```python
from build123d import *

# Parameters (mm, degrees)
SKETCH1_R           = 2.413
BOSS_EXTRUDE1_DEPTH = 3.175
FILLET1_R           = 6.35


with BuildPart() as part:
    # Sketch1 → Boss-Extrude1 (new body)
    with BuildSketch(Plane.XY):
        Polygon((-76.2, 0), (76.2, 0), (76.2, -50.8), (25.4, -50.8), (25.4, -101.6), (-25.4, -101.6), (-25.4, -50.8), (-76.2, -50.8), align=None)
        with Locations((-63.5, -12.7)):
            Circle(SKETCH1_R, mode=Mode.SUBTRACT)
        with Locations((-63.5, -38.1)):
            Circle(SKETCH1_R, mode=Mode.SUBTRACT)
        with Locations((-38.1, -12.7)):
            Circle(SKETCH1_R, mode=Mode.SUBTRACT)
        with Locations((-38.1, -38.1)):
            Circle(SKETCH1_R, mode=Mode.SUBTRACT)
        with Locations((-12.7, -88.9)):
            Circle(SKETCH1_R, mode=Mode.SUBTRACT)
        with Locations((-12.7, -63.5)):
            Circle(SKETCH1_R, mode=Mode.SUBTRACT)
        with Locations(Location((12.7, -88.9, 0), (0, 0, 180))):
            Circle(SKETCH1_R, mode=Mode.SUBTRACT)
        with Locations(Location((12.7, -63.5, 0), (0, 0, 180))):
            Circle(SKETCH1_R, mode=Mode.SUBTRACT)
        with Locations(Location((63.5, -38.1, 0), (0, 0, 180))):
            Circle(SKETCH1_R, mode=Mode.SUBTRACT)
        with Locations(Location((38.1, -38.1, 0), (0, 0, 180))):
            Circle(SKETCH1_R, mode=Mode.SUBTRACT)
        with Locations(Location((38.1, -12.7, 0), (0, 0, 180))):
            Circle(SKETCH1_R, mode=Mode.SUBTRACT)
        with Locations(Location((63.5, -12.7, 0), (0, 0, 180))):
            Circle(SKETCH1_R, mode=Mode.SUBTRACT)
    extrude(amount=BOSS_EXTRUDE1_DEPTH)

    # Fillet1
    fillet1_edges = [part.edges().sort_by_distance(p)[0] for p in [
        (25.4, -101.6, 1.5875),
        (-25.4, -101.6, 1.5875),
        (-25.4, -50.8, 1.5875),
        (-76.2, -50.8, 1.5875),
        (-76.2, 0, 1.5875),
        (76.2, 0, 1.5875),
        (76.2, -50.8, 1.5875),
        (25.4, -50.8, 1.5875),
    ]]
    fillet(fillet1_edges, radius=FILLET1_R)


solid = part.part
```
The model under review builds one solid part; all positions refer to its coordinate system, in mm. A direction names the side the tool comes from. Round coordinates to 2 decimals unless told otherwise and drop trailing zeros. Loops run counter-clockwise (first coordinate to the right, second up) from the corner with the lowest first, then second, coordinate; pieces in that order, holes last. Notation, with made-up numbers: (76, -1.5) -> (108, -1.5) arc R32 ccw to (108, 28.5) -> close; hole circle Ø8 at (24, 89.25). An arc over 180 degrees is marked (long way). Answer in a Markdown table with one row per item.
1) Tool access review of faces 1 (the flat face through (-25.4, -76, 2)), 2 (the cylindrical face through (39.88, -39.73, 1.57)): name each direction out of +Z, -Z, +X, -X, +Y, -Y from which nothing blocks a thin tool from reaching the whole face with its end or side.
Taken from the geometry:
| item | result |
|---|---|
| face 1 | +Z, -Z, -X, -Y |
| face 2 | +Z, -Z |
2) Consider section B-B, the plane z = 1.95. Count the separate pieces of the cut face and the enclosed holes in it, plus the area to 3 significant figures.
Taken from the geometry:
| item | result |
|---|---|
| separate pieces | 1 |
| enclosed holes | 12 |
| area | 10,100 mm² |
3) Draft analysis for pull direction Y (two halves, no side actions). For faces 3 (the cylindrical face through (74.39, -48.89, 1.61)), 4 (the cylindrical face through (65.28, -39.73, 1.57)), 5 (the cylindrical face through (74.29, -1.81, 1.61)), state which applies: pulls with the +Y half, pulls with the -Y half, needs draft (parallel to the pull), parting line crosses it, or undercut.
Taken from the geometry:
| item | result |
|---|---|
| face 3 | pulls with the -Y half |
| face 4 | undercut |
| face 5 | pulls with the +Y half |
4) Consider section A-A, the plane x = 63.5. Write out the cut boundary in (y, z) (3 decimals).
Taken from the geometry:
| item | result |
|---|---|
| outline | (-50.8, 0) -> (-40.513, 0) -> (-40.513, 3.175) -> (-50.8, 3.175) -> close; (-35.687, 0) -> (-15.113, 0) -> (-15.113, 3.175) -> (-35.687, 3.175) -> close; (-10.287, 0) -> (0, 0) -> (0, 3.175) -> (-10.287, 3.175) -> close |
5) Wall thickness on line 1 along Y through (x, z) = (12.7, 1.8); line 2 along Y through (x, z) = (-38.1, 1.8); line 3 along X through (y, z) = (-82.5, 2.2): over which ranges is each line inside the solid? List them lowest first.
Taken from the geometry:
| item | result |
|---|---|
| line 1 | y = -101.6 to -91.31, -86.49 to -65.91, -61.09 to 0 |
| line 2 | y = -50.8 to -40.51, -35.69 to -15.11, -10.29 to 0 |
| line 3 | x = -25.4 to 25.4 |
6) Consider section D-D, the plane y = -75. Write out the cut boundary in (x, z) (3 decimals).
Taken from the geometry:
| item | result |
|---|---|
| outline | (-25.4, 0) -> (25.4, 0) -> (25.4, 3.175) -> (-25.4, 3.175) -> close |
7) For pin 1 Ø1 at (x, z) = (50, 1) entering from -Y, flat-tipped, find the tip position at first contact; note if it passes through.
Taken from the geometry:
| item | result |
|---|---|
| pin 1 | stops at y = -50.8 |
8) Consider section C-C, the plane x = 37.5. Write out the cut boundary in (y, z) (3 decimals).
Taken from the geometry:
| item | result |
|---|---|
| outline | (-50.8, 0) -> (-40.437, 0) -> (-40.437, 3.175) -> (-50.8, 3.175) -> close; (-35.763, 0) -> (-15.037, 0) -> (-15.037, 3.175) -> (-35.763, 3.175) -> close; (-10.363, 0) -> (0, 0) -> (0, 3.175) -> (-10.363, 3.175) -> close |
